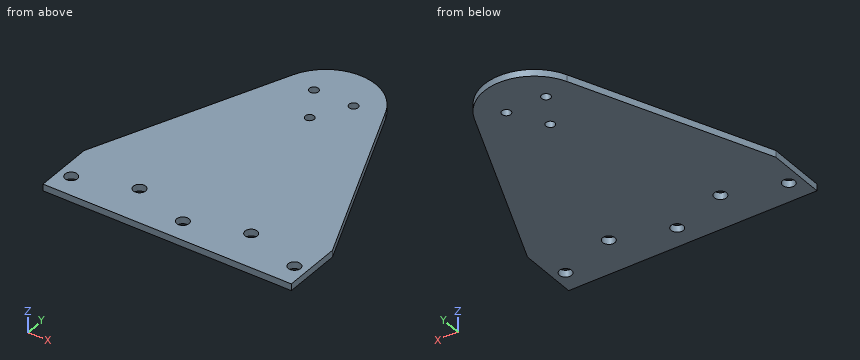
Autodesk Inventor part; units mm, degrees
ref_plane "YZ Plane" through (0, 0, 0) normal (1, 0, 0) x (0, 1, 0)
ref_plane "XZ Plane" through (0, 0, 0) normal (0, 1, 0) x (-1, 0, 0)
ref_plane "XY Plane" through (0, 0, 0) normal (0, 0, 1) x (1, 0, 0)
sketch "Szkic1" plane through (0, 0, 0) normal (0, 0, 1) x (1, 0, 0)
  circle A0 centre (55.6246, 7) radius 2.75
  circle A1 centre (30.6246, 15) radius 2.75
  circle A2 centre (80.6246, 15) radius 2.75
  circle A3 centre (5.6246, 7) radius 2.75
  circle A4 centre (105.6246, 7) radius 2.75
  line L0 (111.2491, 0) -> (0, 0)
  line L1 (111.2491, 0) -> (111.2491, 23.25)
  line L2 (0, 23.25) -> (111.2491, 23.25)
  line L3 (0, 0) -> (0, 23.25)
  line L4 (55.6245, 23.25) -> (55.6245, 98.25)
  circle A5 centre (55.6245, 98.25) radius 22.5
  line L5 (111.2491, 23.25) -> (24.4674, 231.5289)
  line L6 (0, 23.25) -> (68.7685, 188.2966)
  point P0 (76.3938, 106.9037)
  point P1 (34.8553, 106.9037)
  dimension "d0" = 75
  dimension "d1" = 98.25
  dimension "d2" = 45
extrude "Wyciągnięcie proste1" add sketch "Szkic1" along normal blind 3 contours L0 L3 L2 L1 | L2 L4 A5 L5 | L6 A5 L4 L2 | A5
sketch "Szkic2" plane through (0, 0, 3) normal (0, 0, 1) x (1, 0, 0)
  line L0 (34.8553, 106.9037) -> (0, 23.25)
  line L1 (0, 23.25) -> (0, 0)
  line L2 (0, 0) -> (111.2491, 0)
  line L3 (111.2491, 0) -> (111.2491, 23.25)
  line L4 (111.2491, 23.25) -> (76.3938, 106.9037)
  arc A0 (76.3938, 106.9037) -> (34.8553, 106.9037) centre (55.6245, 98.25) ccw
  circle A1 centre (105.6246, 7) radius 2.75
  circle A2 centre (5.6246, 7) radius 2.75
  circle A3 centre (80.6246, 15) radius 2.75
  circle A4 centre (30.6246, 15) radius 2.75
  circle A5 centre (55.6246, 7) radius 2.75
  line L5 (55.6245, 98.25) -> (55.6245, 88)
  circle A6 centre (55.6245, 88) radius 2
  circle A7 centre (64.5013, 103.375) radius 2
  circle A8 centre (46.7478, 103.375) radius 2
  dimension "d5" = 10.25
  dimension "d6" = 4
  dimension "d9" = 360
extrude "Wyciągnięcie proste2" cut sketch "Szkic2" against normal through all contours A6 | A7 | A8
move faces "Przesuń1" translate (0, -3, 0) faces at (37.083, 0, 1)
properties part number "BLACHA_2_Przegub" material "Aluminium 6061"
Check sheet for the modelled part. Datum: model origin and axes. Units: mm. Coordinates: 2 decimals unless noted, no trailing zeros. Loops run counter-clockwise (first coordinate to the right, second up) from the corner with the lowest first, then second, coordinate; pieces in that order, holes last.
1) Sectioned sample at B-B (x = 47). Record the boundary of the cut face in (y, z).
2) Gauge pin test, flat ends, axial feed: pin 1 (1.5 mm diameter, centred on y = 89.5, z = 0.5, fed in from -X); pin 2 (4.5 mm diameter, centred on x = 80.62, y = 15, fed in from -Z). Record the tip position at first contact, or that the pin passes through.
3) Sectioned sample at C-C (y = 88). Record the boundary of the cut face in (x, z).
4) Sectioned sample at D-D (z = 0.65). Count the separate pieces of the cut face and the enclosed holes in it, and give its area (3 significant figures).
5) Material ranges on probe 1 along X at (y, z) = (7, 1.5); probe 2 along X at (y, z) = (105, 0.9); probe 3 along X at (y, z) = (87, 0.9), recorded low to high.
6) Sectioned sample at A-A (y = 7). Record the boundary of the cut face in (x, z), and give its area (3 significant figures).
Check sheet entries:
1. outline: (-3, 0) - (101.39, 0) - (101.39, 3) - (-3, 3) - close; (105.36, 0) - (119.03, 0) - (119.03, 3) - (105.36, 3) - close
2. pin 1: stops at x = 27.29
2. pin 2: passes through
3. outline: (26.98, 0) - (53.62, 0) - (53.62, 3) - (26.98, 3) - close; (57.62, 0) - (84.27, 0) - (84.27, 3) - (57.62, 3) - close
4. separate pieces: 1
4. enclosed holes: 8
4. area: 9,570 mm2
5. probe 1: x = 0 to 2.87, 8.37 to 52.87, 58.37 to 102.87, 108.37 to 111.25
5. probe 2: x = 34.06 to 45.58, 47.91 to 63.34, 65.67 to 77.19
5. probe 3: x = 26.56 to 53.89, 57.36 to 84.69
6. outline: (0, 0) - (2.87, 0) - (2.87, 3) - (0, 3) - close; (8.37, 0) - (52.87, 0) - (52.87, 3) - (8.37, 3) - close; (58.37, 0) - (102.87, 0) - (102.87, 3) - (58.37, 3) - close; (108.37, 0) - (111.25, 0) - (111.25, 3) - (108.37, 3) - close
6. area: 284 mm2
